Check sheet for the modelled part. Datum: model origin and axes. Units: mm. A direction names the side the tool comes from. Give positions to 0.01 mm unless a question says otherwise; leave off trailing zeros. Loops run counter-clockwise (first coordinate to the right, second up) from the corner with the lowest first, then second, coordinate; pieces in that order, holes last. Notation, with made-up numbers: (24.5, 1) - (50.5, 1) arc R36 cw to (50.5, 35) - close; hole circle Ø5 at (36, 67). An arc over 180 degrees is marked (long way). Answer in a Markdown table with one row per item. Add a question column.
(1) Sectioned sample at B-B on x = -118. Enter the section's corners in (y, z), then the cut area to 3 significant figures.
(2) Draft check along X on faces 4 (the face through (-200, -10, -97)), 5 (the face through (3.2, -320.1, -170.1)), 6 (the face through (-43.139, -555.732, -202.465)), 7 (the face through (-3, 499, 0)). Enter one of: released by +X, released by -X, zero draft, split by the parting line, or undercut.
(3) Sectioned sample at D-D on y = -651. Enter the section's corners in (x, z), then the cut area to 3 significant figures.
(4) Thickness scan on L1, parallel to Y at x = 8.5, z = -90; L2, parallel to Y at x = 120.5, z = -65.5; L3, parallel to Z at x = 137, y = -844. Record the ranges inside material, lowest first.
(5) Sectioned sample at C-C on z = 111. Enter the section's corners in (x, y).
(6) Go/stop test with flat-tipped pins: P1, Ø12, axis at x = 88.5, z = -140.5, coming from the +Y side; P2, Ø2, axis at x = -92, z = -210, coming from the +Y side. Record where each tip stops, or that it passes through.
(7) Sectioned sample at A-A on y = 463. Enter the section's corners in (x, z).
(8) Set-up check for faces 1 (the face through (-3, -561, 0)), 2 (the face through (200, 10, -97)), 3 (the face through (-3, -753, -205)): record each of +Z, -Z, +X, -X, +Y, -Y from which the full face is reachable in a straight line by a thin tool's end or side.
from build123d import *

# Parameters (mm, degrees)
F0_W     = 400
F0_H     = 1500
F1_DEPTH = 145
F2_R     = 177.5
F3_DEPTH = 200
F5_DEPTH = 145
F6_R     = 199
F7_DEPTH = 5


with BuildPart() as f1:
    # F0 (on Top) → F1 (new body)
    with BuildSketch(Plane.XY):
        with BuildLine():
            ThreePointArc((200, 750), (0, 950), (-200, 750))
            Line((-200, 750), (200, 750))
        make_face()
        Rectangle(F0_W, F0_H)
        with BuildLine():
            Line((200, -750), (-200, -750))
            ThreePointArc((-200, -750), (0, -950), (200, -750))
        make_face()
    extrude(amount=F1_DEPTH)

    # F2 (on face) → F3 (join)
    with BuildSketch(Plane(origin=(0, 0, 0), x_dir=(1, 0, 0), z_dir=(0, 0, -1))):
        with Locations((0, 750)):
            Circle(F2_R)
        with Locations((0, -750)):
            Circle(F2_R)
        with BuildLine():
            ThreePointArc((200, 404.203802), (0.034243, 320.081481), (-200, 404.040821))
            Line((-200, 404.040821), (-200, -404.040821))
            ThreePointArc((-200, -404.040821), (0, -320), (200, -404.040821))
            Line((200, -404.040821), (200, 404.203802))
        make_face()
    extrude(amount=F3_DEPTH)

    # F4 (on face) → F5 (join)
    with BuildSketch(Plane(origin=(0, 0, -200), x_dir=(1, 0, 0), z_dir=(0, 0, -1))):
        with BuildLine():
            Line((-200, 404.040821), (-200, -750))
            Line((-200, -750), (200, -750))
            Line((200, -750), (200, 404.203802))
            ThreePointArc((200, 404.203802), (0.034243, 320.081481), (-200, 404.040821))
        make_face()
        with BuildLine():
            Line((200, -750), (-200, -750))
            ThreePointArc((-200, -750), (0, -950), (200, -750))
        make_face()
    extrude(amount=F5_DEPTH)

    # F6 (on face) → F7 (join)
    with BuildSketch(Plane(origin=(0, 0, -200), x_dir=(1, 0, 0), z_dir=(0, 0, -1))):
        with Locations((0, 750)):
            Circle(F6_R)
    extrude(amount=F7_DEPTH)


solid = f1.part
Reply:
| question | item | result |
|---|---|---|
| 1 | outline | (-911.48, 0) - (-882.6, 0) - (-882.6, -200) - (-910.24, -200) - (-910.24, -205) - (-589.76, -205) - (-589.76, -200) - (-617.4, -200) - (-617.4, 0) - (-346.12, 0) - (-346.12, -345) - (911.48, -345) - (911.48, -200) - (882.6, -200) - (882.6, 0) - (911.48, 0) - (911.48, 145) - (-911.48, 145) - close; hole (346.08, -200) - (617.4, -200) - (617.4, 0) - (346.08, 0) - close |
| 1 | area | 693,000 mm^2 |
| 2 | face 4 | released by -X |
| 2 | face 5 | undercut |
| 2 | face 6 | split by the parting line |
| 2 | face 7 | undercut |
| 3 | outline | (-200, 0) - (-147.33, 0) - (-147.33, -200) - (-172.63, -200) - (-172.63, -205) - (172.63, -205) - (172.63, -200) - (147.33, -200) - (147.33, 0) - (200, 0) - (200, 145) - (-200, 145) - close |
| 3 | area | 119,000 mm^2 |
| 4 | L1 | -927.3 to -572.7, -320.21 to 320.13, 572.7 to 927.3 |
| 4 | L2 | -880.33 to -619.67, -347.38 to 347.26, 619.67 to 880.33 |
| 4 | L3 | -205 to 145 |
| 5 | outline | (-200, -750) arc R200 ccw to (200, -750) - (200, 750) arc R200 ccw to (-200, 750) - close |
| 6 | P1 | y = 907.16 |
| 6 | P2 | y = 928.1 |
| 7 | outline | (-200, -345) - (200, -345) - (200, -200) - (-200, -200) - close; (-200, 0) - (200, 0) - (200, 145) - (-200, 145) - close |
| 8 | face 1 | none |
| 8 | face 2 | +Z, -Z, +X, +Y, -Y |
| 8 | face 3 | -Z, +X, -X, -Y |
